Read the model definition and answer for the solid it produces. Units are mm, in the model's axes. Coordinates: 2 decimals unless noted, no trailing zeros. Loops run counter-clockwise (first coordinate to the right, second up) from the corner with the lowest first, then second, coordinate; pieces in that order, holes last. Notation, with made-up numbers: (35, 8) - (42, 8) arc R29 ccw to (42, 31) - close; hole circle Ø10 at (29, -39.75). An arc over 180 degrees is marked (long way). One line per item, written item: value. Start each with the question number.
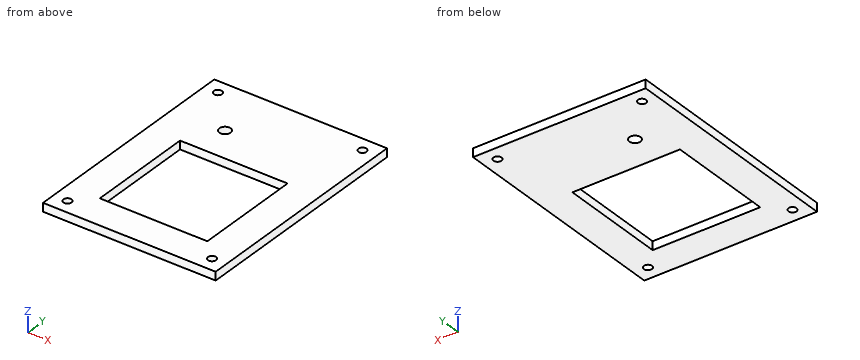
Autodesk Fusion 360 part; units mm, degrees
sketch "Sketch1" plane through (0, 0, 0) normal (0, 0, 1) x (1, 0, 0)
  line L0 (0, 0) -> (61.5, 0)
  line L1 (61.5, 0) -> (61.5, 82)
  line L2 (61.5, 82) -> (0, 82)
  line L3 (0, 82) -> (0, 0)
  dimension "d1" = 82
  dimension "d2" = 61.5
extrude "Extrude1" add sketch "Sketch1" along normal blind 3
sketch "Sketch2" plane through (0, 0, 3) normal (0, 0, 1) x (-1, 0, 0)
  line L0 (0, -82) -> (0, 0)
  line L1 (0, 0) -> (-61.5, 0)
  line L2 (-61.5, 0) -> (-61.5, -82)
  line L3 (-61.5, -82) -> (0, -82)
  circle A0 centre (-5, -5) radius 1.45
  circle A1 centre (-5, -77) radius 1.45
  circle A2 centre (-56.5, -77) radius 1.45
  circle A3 centre (-56.5, -5) radius 1.45
  dimension "d5" = 2.9
  dimension "d6" = 5
  dimension "d7" = 5
  dimension "d8" = 2.9
  dimension "d9" = 5
  dimension "d10" = 5
  dimension "d11" = 2.9
  dimension "d12" = 5
  dimension "d13" = 5
  dimension "d14" = 2.9
  dimension "d15" = 5
  dimension "d16" = 5
extrude "Extrude2" cut sketch "Sketch2" against normal blind 3 contours A0 | A1 | A2 | A3
sketch "Sketch3" plane through (0, 0, 0) normal (0, 0, 1) x (1, 0, 0)
  line L0 (10, 72) -> (51.5, 72)
  line L1 (51.5, 72) -> (51.5, 10)
  line L2 (51.5, 10) -> (10, 10)
  line L3 (10, 10) -> (10, 72)
  line L4 (61.5, 82) -> (0, 82)
  line L5 (61.5, 0) -> (61.5, 82)
  line L6 (0, 0) -> (61.5, 0)
  line L7 (0, 82) -> (0, 0)
  dimension "d19" = 10
  dimension "d20" = 10
  dimension "d21" = 10
  dimension "d22" = 10
sketch "Sketch4" plane through (0, 0, 0) normal (0, 0, 1) x (1, 0, 0)
sketch "Sketch5" plane through (0, 0, 0) normal (0, 0, 1) x (1, 0, 0)
sketch "Sketch6" plane through (0, 0, 0) normal (0, 0, 1) x (1, 0, 0)
  line L0 (49.9, 50) -> (11.6, 50)
  line L1 (11.6, 50) -> (11.6, 11.6)
  line L2 (11.6, 11.6) -> (49.9, 11.6)
  line L3 (49.9, 11.6) -> (49.9, 50)
  line L4 (51.5, 72) -> (51.5, 10)
  line L5 (10, 10) -> (10, 72)
  line L6 (51.5, 10) -> (10, 10)
  line L7 (10, 72) -> (51.5, 72)
  dimension "d23" = 1.6
  dimension "d24" = 1.6
  dimension "d25" = 1.6
  dimension "d26" = 22
sketch "Sketch7" plane through (0, 0, 0) normal (0, 0, 1) x (1, 0, 0)
  circle A0 centre (18.7, 62) radius 2
  line L0 (10, 72) -> (51.5, 72)
  line L1 (10, 10) -> (10, 72)
  dimension "d30" = 4
  dimension "d31" = 10
  dimension "d32" = 8.7
extrude "Extrude3" cut sketch "Sketch6" sketch "Sketch7" along normal blind 3 contours L0 L1 L2 L3 of sketch 2
1) Section B-B, the plane x = 46.5 is taken. Determine the outline of the cut face in (y, z).
2) Straight lines are drawn through the part: L1, parallel to X at y = 5, z = 2.2; L2, parallel to Y at x = 56.5, z = 1.45; L3, parallel to X at y = 25, z = 1.15. For each, find the intervals that lie inside material, in ascending order.
3) Section C-C, the plane x = 5 is taken. Determine the outline of the cut face in (y, z).
4) Section D-D, the plane z = 0.75 is taken. Determine the outline of the cut face in (x, y), and give its area (3 significant figures).
5) Section A-A, the plane y = 23 is taken. Determine the outline of the cut face in (x, z).
Answer below:
1. outline: (0, 0) - (11.6, 0) - (11.6, 3) - (0, 3) - close; (50, 0) - (82, 0) - (82, 3) - (50, 3) - close
2. L1: 0 to 3.55, 6.45 to 55.05, 57.95 to 61.5
2. L2: 0 to 3.55, 6.45 to 75.55, 78.45 to 82
2. L3: 0 to 11.6, 49.9 to 61.5
3. outline: (0, 0) - (3.55, 0) - (3.55, 3) - (0, 3) - close; (6.45, 0) - (75.55, 0) - (75.55, 3) - (6.45, 3) - close; (78.45, 0) - (82, 0) - (82, 3) - (78.45, 3) - close
4. outline: (0, 0) - (61.5, 0) - (61.5, 82) - (0, 82) - close; hole circle Ø2.9 at (5, 5); hole circle Ø2.9 at (5, 77); hole (11.6, 11.6) - (49.9, 11.6) - (49.9, 50) - (11.6, 50) - close; hole circle Ø4 at (18.7, 62); hole circle Ø2.9 at (56.5, 5); hole circle Ø2.9 at (56.5, 77)
4. area: 3,530 mm2
5. outline: (0, 0) - (11.6, 0) - (11.6, 3) - (0, 3) - close; (49.9, 0) - (61.5, 0) - (61.5, 3) - (49.9, 3) - close
